Check sheet for the modelled part. Datum: model origin and axes. Units: mm. Face numbers are marked on the shaded views. A direction names the side the tool comes from. Give positions to 0.01 mm unless a question says otherwise; leave off trailing zeros. Write each loop counter-clockwise with the first axis right and the second up, starting at its lowest first coordinate (ties: lowest second). Pieces come first, ordered by that corner, then holes.
from build123d import *

# Parameters (mm, degrees)
CYLINDER087_R           = 1.3
CYLINDER087_DEPTH       = 40
CYLINDER087_PITCH_ANGLE = 90
CYLINDER086_R           = 1.3
CYLINDER086_DEPTH       = 40
CYLINDER086_PITCH_ANGLE = 90
CYLINDER085_R           = 1.3
CYLINDER085_DEPTH       = 40
CYLINDER085_PITCH_ANGLE = 90
CYLINDER067_R           = 1.8
CYLINDER067_DEPTH       = 40
BOX034_W                = 4
BOX034_H                = 16
BOX034_DEPTH            = 10
BOX031_W                = 8
BOX031_H                = 34
BOX031_DEPTH            = 4
BOX033_W                = 6
BOX033_H                = 16
BOX033_DEPTH            = 10
CHAMFER008_SIZE         = 4


with BuildPart() as cylinder365:
    # Cylinder087 → Cylinder087 (new body)
    with BuildSketch(Plane.XY):
        Circle(CYLINDER087_R)
    extrude(amount=CYLINDER087_DEPTH)


with BuildPart() as cylinder365_1:
    # Cylinder087 pitch: moved
    add(cylinder365.part.rotate(Axis((0, 0, 0), (0, 1, 0)), CYLINDER087_PITCH_ANGLE))


with BuildPart() as cylinder365_2:
    # Cylinder087 placement: moved
    add(cylinder365_1.part.moved(Location((-48, 7, 30))))


with BuildPart() as cylinder364:
    # Cylinder086 → Cylinder086 (new body)
    with BuildSketch(Plane.XY):
        Circle(CYLINDER086_R)
    extrude(amount=CYLINDER086_DEPTH)


with BuildPart() as cylinder364_1:
    # Cylinder086 pitch: moved
    add(cylinder364.part.rotate(Axis((0, 0, 0), (0, 1, 0)), CYLINDER086_PITCH_ANGLE))


with BuildPart() as cylinder364_2:
    # Cylinder086 placement: moved
    add(cylinder364_1.part.moved(Location((-67, -15, 30))))


with BuildPart() as hinge_screw_holes_b003:
    # Cylinder085 → Cylinder085 (new body)
    with BuildSketch(Plane.XY):
        Circle(CYLINDER085_R)
    extrude(amount=CYLINDER085_DEPTH)


with BuildPart() as hinge_screw_holes_b003_1:
    # Cylinder085 pitch: moved
    add(hinge_screw_holes_b003.part.rotate(Axis((0, 0, 0), (0, 1, 0)), CYLINDER085_PITCH_ANGLE))


with BuildPart() as hinge_screw_holes_b003_2:
    # Cylinder085 placement: moved
    add(hinge_screw_holes_b003_1.part.moved(Location((-92, -7, 30))))

    # Fusion057: union Cylinder364
    add(cylinder364_2.part)

    # Fusion058: union Cylinder365
    add(cylinder365_2.part)


with BuildPart() as cylinder345:
    # Cylinder067 → Cylinder067 (new body)
    with BuildSketch(Plane(origin=(-56, 7, 15), x_dir=(1, 0, 0), z_dir=(0, 0, 1))):
        Circle(CYLINDER067_R)
    extrude(amount=CYLINDER067_DEPTH)


with BuildPart() as cube022:
    # Box034 → Box034 (new body)
    with BuildSketch(Plane(origin=(-54, -19, 25), x_dir=(1, 0, 0), z_dir=(0, 0, 1))):
        with Locations((2, 8)):
            Rectangle(BOX034_W, BOX034_H)
    extrude(amount=BOX034_DEPTH)


with BuildPart() as cut038:
    # Box031 → Box031 (new body)
    with BuildSketch(Plane(origin=(-60, -19, 28), x_dir=(1, 0, 0), z_dir=(0, 0, 1))):
        with Locations((4, 17)):
            Rectangle(BOX031_W, BOX031_H)
    extrude(amount=BOX031_DEPTH)

    # Cut038: cut Cube022
    add(cube022.part, mode=Mode.SUBTRACT)


with BuildPart() as switch_rocker_f:
    # Box033 → Box033 (new body)
    with BuildSketch(Plane(origin=(-60, -19, 25), x_dir=(1, 0, 0), z_dir=(0, 0, 1))):
        with Locations((3, 8)):
            Rectangle(BOX033_W, BOX033_H)
    extrude(amount=BOX033_DEPTH)

    # Fusion044: union Cut038
    add(cut038.part)

    # Cut039: cut Cylinder345
    add(cylinder345.part, mode=Mode.SUBTRACT)

    # Cut047: cut hinge-screw-holes-b003
    add(hinge_screw_holes_b003_2.part, mode=Mode.SUBTRACT)

    # Chamfer008
    chamfer008_edges = [switch_rocker_f.edges().sort_by_distance(p)[0] for p in [
        (-60, 15, 30),
    ]]
    chamfer(chamfer008_edges, length=CHAMFER008_SIZE)


solid = switch_rocker_f.part
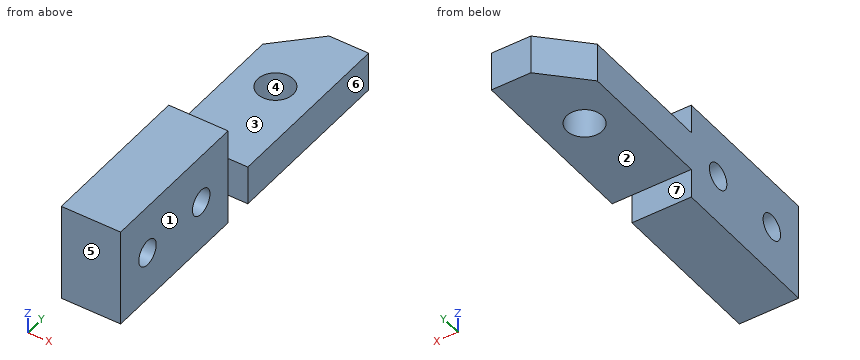
1) Sectioned sample at D-D on z = 27. Record the boundary of the cut face in (x, y).
2) Sectioned sample at C-C on y = -15. Record the boundary of the cut face in (x, z).
3) Sectioned sample at A-A on y = 7. Record the boundary of the cut face in (x, z), then the cut area to 3 significant figures.
4) Access from +Z, -Z, +X, -X, +Y, -Y to the whole of each face (thin tool, end or side, straight path). Record for the marked faces 1, 2 and 3.
5) Draft check along Y on the marked faces 4, 5, 6 and 7. Enter one of: +Y half, -Y half, draft (parallel to the pull), parting line (faces both ways), or undercut.
6) Gauge pin test, flat ends, axial feed: pin 1 (2 mm diameter, centred on x = -53, y = 8.5, fed in from +Z); pin 2 (2.5 mm diameter, centred on x = -56, z = 26, fed in from +Y); pin 3 (3 mm diameter, centred on x = -53.5, y = 4, fed in from -Z); pin 4 (1 mm diameter, centred on y = -0.5, z = 26.5, fed in from -X). Record the tip position at first contact, or that the pin passes through.
7) Sectioned sample at B-B on x = -56.5. Record the boundary of the cut face in (y, z), then the cut area to 3 significant figures.
8) Scan lines: L1, parallel to Y at x = -56, z = 30; L2, parallel to Z at x = -56.35, y = -7; L3, parallel to Y at x = -59.5, z = 29.75. Record each from-to range of solid material in increasing order.
Answers below:
1. outline: (-60, -19) - (-54, -19) - (-54, -3) - (-60, -3) - close
2. outline: (-60, 25) - (-54, 25) - (-54, 28.7) - (-60, 28.7) - close; (-60, 31.3) - (-54, 31.3) - (-54, 35) - (-60, 35) - close
3. outline: (-60, 28) - (-57.8, 28) - (-57.8, 32) - (-60, 32) - close; (-54.2, 28) - (-52, 28) - (-52, 32) - (-54.2, 32) - close
3. area: 17.6 mm2
4. face 1: +Z, -Z, +X, -Y
4. face 2: -Z, +X, -X, +Y
4. face 3: +Z, +X, -X, +Y
5. face 4: undercut
5. face 5: -Y half
5. face 6: draft
5. face 7: +Y half
6. pin 1: stops at z = 32
6. pin 2: stops at y = -3
6. pin 3: stops at z = 28
6. pin 4: passes through
7. outline: (-19, 25) - (-3, 25) - (-3, 28) - (5.27, 28) - (5.27, 32) - (-3, 32) - (-3, 35) - (-19, 35) - close; (8.73, 28) - (14.5, 28) - (14.5, 32) - (8.73, 32) - close; hole circle Ø2.6 at (-15, 30); hole circle Ø2.6 at (-7, 30)
7. area: 206 mm2
8. L1: y = -19 to -16.3, -13.7 to -8.3, -5.7 to 5.2, 8.8 to 15
8. L2: z = 25 to 28.7, 31.3 to 35
8. L3: y = -19 to -16.28, -13.72 to -8.28, -5.72 to 11.5
